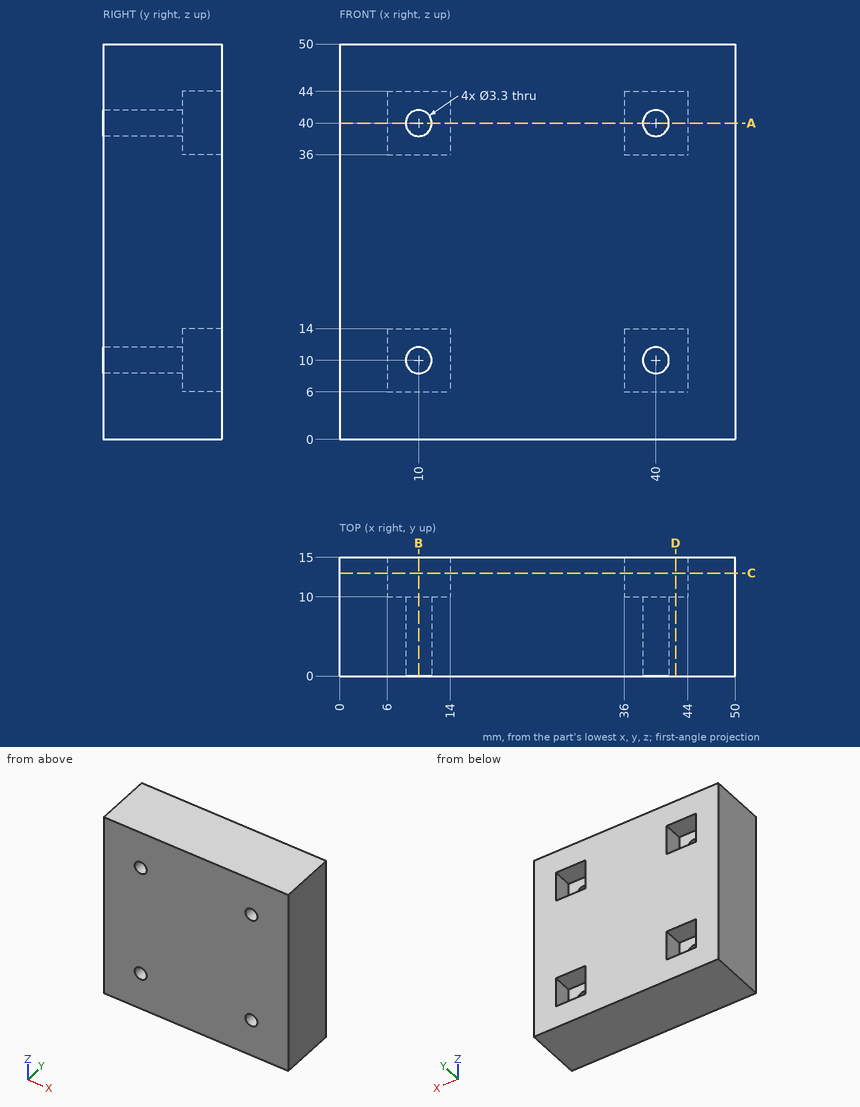
Part print with two shaded views. Sizes in mm from the minimum x, y, z corner. Coordinates: 2 decimals unless noted, no trailing zeros. Order: outer loops, then holes, each group sorted by start corner. A loop starts at its lowest first (then second) coordinate and runs counter-clockwise, first axis right, second up. Notation, with made-up numbers: M 9.25,-38.5 L 53.25,-38.5 A34 cw 53.25,-3.5 Z; hole C 30,75.5 d5. An arc over 180 degrees is marked long. Use a Markdown table: item, result.
(1) Cut at B-B on x = 10. Write the cut outline in (y, z).
A:
| item | result |
|---|---|
| outline | M 0,0 L 15,0 L 15,6 L 10,6 L 10,8.35 L 0,8.35 Z; M 0,11.65 L 10,11.65 L 10,14 L 15,14 L 15,36 L 10,36 L 10,38.35 L 0,38.35 Z; M 0,41.65 L 10,41.65 L 10,44 L 15,44 L 15,50 L 0,50 Z |
(2) Flat gauge pin, fed straight in: pin 1 (1.5 mm diameter, centred on x = 9.5, z = 43, fed in from +Y). Where does the tip first touch, or does it go through?
A:
| item | result |
|---|---|
| pin 1 | stops at y = 10 |
(3) Cut at D-D on x = 42.5. Write the cut outline in (y, z).
A:
| item | result |
|---|---|
| outline | M 0,0 L 15,0 L 15,6 L 10,6 L 10,14 L 15,14 L 15,36 L 10,36 L 10,44 L 15,44 L 15,50 L 0,50 Z |
(4) Cut at C-C on y = 13. Write the cut outline in (x, z), then the cut area to 3 significant figures.
A:
| item | result |
|---|---|
| outline | M 0,0 L 50,0 L 50,50 L 0,50 Z; hole M 6,6 L 14,6 L 14,14 L 6,14 Z; hole M 6,36 L 14,36 L 14,44 L 6,44 Z; hole M 36,6 L 44,6 L 44,14 L 36,14 Z; hole M 36,36 L 44,36 L 44,44 L 36,44 Z |
| area | 2,240 mm^2 |
(5) Probe L1, parallel to X at y = 8, z = 40; L2, parallel to Z at x = 43, y = 12.25. List the from-to ranges inside material, lowest first.
A:
| item | result |
|---|---|
| L1 | x = 0 to 8.35, 11.65 to 38.35, 41.65 to 50 |
| L2 | z = 0 to 6, 14 to 36, 44 to 50 |
(6) Cut at A-A on z = 40. Write the cut outline in (x, y).
A:
| item | result |
|---|---|
| outline | M 0,0 L 8.35,0 L 8.35,10 L 6,10 L 6,15 L 0,15 Z; M 11.65,0 L 38.35,0 L 38.35,10 L 36,10 L 36,15 L 14,15 L 14,10 L 11.65,10 Z; M 41.65,0 L 50,0 L 50,15 L 44,15 L 44,10 L 41.65,10 Z |
